```python
from build123d import *
from build123d.topology import SkipClean

# Parameters (mm, degrees)
BOSS_EXTRUDE1_DEPTH                      = 3
MIRROR1_AT_THE_SECOND_PLANE_COPY_1_DEPTH = 3
SKETCH2_R                                = 1.6
CUT_EXTRUDE1_DEPTH                       = 108.522090753
CHAMFER1_SIZE                            = 1.5
CIRPATTERN1_COUNT                        = 6
CHAMFER1_OF_CIRPATTERN1_SIZE             = 1.5
SKETCH3_R                                = 5
CUT_EXTRUDE2_DEPTH                       = 108.522090753


with BuildPart() as part:
    # Sketch1 → Boss-Extrude1 (new body)
    with BuildSketch(Plane(origin=(0, 0, 0), x_dir=(1, 0, 0), z_dir=(0, 1, 0))):
        with BuildLine():
            Line((-76, -76), (-59.111111111, -76))
            Line((-59.111111111, -76), (-59.111111111, -73))
            Line((-59.111111111, -73), (-42.222222222, -73))
            Line((-42.222222222, -73), (-42.222222222, -76))
            Line((-42.222222222, -76), (-25.333333333, -76))
            Line((-25.333333333, -76), (-25.333333333, -73))
            Line((-25.333333333, -73), (-8.444444444, -73))
            Line((-8.444444444, -73), (-8.444444444, -76))
            Line((-8.444444444, -76), (0, -76))
            Line((0, -76), (0, -10.5))
            ThreePointArc((0, -10.5), (-7.424621202, -7.424621202), (-10.5, 0))
            Line((-10.5, 0), (-76, 0))
            Line((-76, 0), (-76, -8.444444444))
            Line((-76, -8.444444444), (-73, -8.444444444))
            Line((-73, -8.444444444), (-73, -25.333333333))
            Line((-73, -25.333333333), (-76, -25.333333333))
            Line((-76, -25.333333333), (-76, -42.222222222))
            Line((-76, -42.222222222), (-73, -42.222222222))
            Line((-73, -42.222222222), (-73, -59.111111111))
            Line((-73, -59.111111111), (-76, -59.111111111))
            Line((-76, -59.111111111), (-76, -76))
        make_face()
    boss_extrude1 = extrude(amount=BOSS_EXTRUDE1_DEPTH)

    # Mirror1 at the second plane: Boss-Extrude1 across plane
    add(boss_extrude1.mirror(Plane(origin=(0, 0, 0), x_dir=(0, 0, 1), z_dir=(1, 0, 0))))



with BuildPart() as mirror1_1:
    # Mirror1: Boss-Extrude1 across plane
    add(boss_extrude1.mirror(Plane.XY))


with BuildPart() as part_1:
    with SkipClean():  # the faces are left unmerged after this step: merging them gives an invalid solid
        add(part.part)

        add(mirror1_1.part)  # Mirror1 at the second plane copy 1 merges Mirror1_1
        # Mirror1 at the second plane copy 1 sketc → Mirror1 at the second plane copy 1 (add)
        with BuildSketch(Plane(origin=(0, 0, 0), x_dir=(-1, 0, 0), z_dir=(0, 1, 0))):
            with BuildLine():
                Line((-76, -76), (-59.111111111, -76))
                Line((-59.111111111, -76), (-59.111111111, -73))
                Line((-59.111111111, -73), (-42.222222222, -73))
                Line((-42.222222222, -73), (-42.222222222, -76))
                Line((-42.222222222, -76), (-25.333333333, -76))
                Line((-25.333333333, -76), (-25.333333333, -73))
                Line((-25.333333333, -73), (-8.444444444, -73))
                Line((-8.444444444, -73), (-8.444444444, -76))
                Line((-8.444444444, -76), (0, -76))
                Line((0, -76), (0, -10.5))
                ThreePointArc((0, -10.5), (-7.424621202, -7.424621202), (-10.5, 0))
                Line((-10.5, 0), (-76, 0))
                Line((-76, 0), (-76, -8.444444444))
                Line((-76, -8.444444444), (-73, -8.444444444))
                Line((-73, -8.444444444), (-73, -25.333333333))
                Line((-73, -25.333333333), (-76, -25.333333333))
                Line((-76, -25.333333333), (-76, -42.222222222))
                Line((-76, -42.222222222), (-73, -42.222222222))
                Line((-73, -42.222222222), (-73, -59.111111111))
                Line((-73, -59.111111111), (-76, -59.111111111))
                Line((-76, -59.111111111), (-76, -76))
            make_face()
        extrude(amount=MIRROR1_AT_THE_SECOND_PLANE_COPY_1_DEPTH)

    # Sketch2 → Cut-Extrude1 (cut, through all)
    with SkipClean():  # the faces are left unmerged after this step: merging them gives an invalid solid
        with BuildSketch(Plane(origin=(0, 3, 0), x_dir=(1, 0, 0), z_dir=(0, 1, 0))):
            with Locations(Location((0, 21, 0), (0, 0, 270))):
                Circle(SKETCH2_R)
        cut_extrude1 = extrude(amount=-CUT_EXTRUDE1_DEPTH, mode=Mode.SUBTRACT)

    # Chamfer1
    chamfer1_edges = [part_1.edges().sort_by_distance(p)[0] for p in [
        (-1.6, 0, -21),
    ]]
    chamfer(chamfer1_edges, length=CHAMFER1_SIZE)

    # CirPattern1: Cut-Extrude1 ×6 about axis
    cirpattern1_axis = Axis((0, 0, 0), (0, 1, 0))
    for i in range(1, CIRPATTERN1_COUNT):
        add(cut_extrude1.rotate(cirpattern1_axis, i * 360 / CIRPATTERN1_COUNT), mode=Mode.SUBTRACT)

    # Chamfer1 of CirPattern1
    chamfer1_of_cirpattern1_edges = [part_1.edges().sort_by_distance(p)[0] for p in [
        (-18.986533479, 0, -9.114359354),
        (-17.386533479, 0, 11.885640646),
        (1.6, 0, 21),
        (18.986533479, 0, 9.114359354),
        (17.386533479, 0, -11.885640646),
    ]]
    chamfer(chamfer1_of_cirpattern1_edges, length=CHAMFER1_OF_CIRPATTERN1_SIZE)

    # Sketch3 → Cut-Extrude2 (cut, through all)
    with BuildSketch(Plane(origin=(0, 3, 0), x_dir=(1, 0, 0), z_dir=(0, 1, 0))):
        with Locations(Location((0, 42.5, 0), (0, 0, 270))):
            Circle(SKETCH3_R)
        with BuildLine():
            ThreePointArc((-21.372688022, 25.470977734), (-21.865715356, 19.835649522), (-16.230387145, 19.342622189))
            ThreePointArc((-16.230387145, 19.342622189), (0, 25.25), (16.230387145, 19.342622189))
            ThreePointArc((16.230387145, 19.342622189), (21.865715356, 19.835649522), (21.372688022, 25.470977734))
            ThreePointArc((21.372688022, 25.470977734), (0, 33.25), (-21.372688022, 25.470977734))
        make_face()
    cut_extrude2 = extrude(amount=-CUT_EXTRUDE2_DEPTH, mode=Mode.SUBTRACT)

    # Mirror2: Cut-Extrude2 across plane
    add(cut_extrude2.mirror(Plane.XY), mode=Mode.SUBTRACT)


solid = part_1.part
```
The model under review builds one solid part; all positions refer to its coordinate system, in mm. A direction names the side the tool comes from. Round coordinates to 2 decimals unless told otherwise and drop trailing zeros. Loops run counter-clockwise (first coordinate to the right, second up) from the corner with the lowest first, then second, coordinate; pieces in that order, holes last. Notation, with made-up numbers: (53.25, 11.25) -> (81.25, 11.25) arc R19 cw to (81.25, 27.25) -> close; hole circle Ø9 at (46, 72). An arc over 180 degrees is marked (long way). Answer as a JSON object with one key per item and string values. Group by question number.
1) We need section C-C on y = 2. Give the number of separate pieces and of enclosed holes in the cut face, then the cut area to 3 significant figures.
2) For faces 1 (the face through (-0.25, 1.52, 25.25)), 2 (the face through (1, 3, 18)), list the 3-axis set-ups (+Z, -Z, +X, -X, +Y, -Y) from which the entire face can be reached by the end or side of a thin tool; tool diameter is ignored.
3) We need section B-B on z = 16. Write out the cut boundary in (x, y), then the cut area to 3 significant figures.
4) Mouldability with a two-part tool opening along X and no side actions: class faces 3 (the face through (-21.92, 1.52, -19.9)), 4 (the face through (18, 0, 1)) as released by +X, released by -X, zero draft, split by the parting line, or undercut.
5) For line 1 (Z direction, x = -12, y = 1.95); line 2 (Z direction, x = 17, y = 2.3); line 3 (X direction, y = 2.2, z = 21), list the stretches that pass through material, from the lowest coordinate up. Write a range as [from, to].
6) We need section A-A on z = -44. Write out the cut boundary in (x, y), then the cut area to 3 significant figures.
7) For pin 1 Ø0.9 at (x, y) = (17, 2) entering from +Z; pin 2 Ø1 at (y, z) = (2.5, 51) entering from +X; pin 3 Ø1.9 at (x, z) = (18.19, 10.5) entering from +Y; pin 4 Ø0.9 at (y, z) = (2, -17.5) entering from -X, all flat-tipped, find the tip position at first contact; note any pin that passes through.
Result set:
{
 "1": {"separate pieces": "1", "enclosed holes": "11", "area": "21,000 mm²"},
 "2": {"face 1": "+Y, -Y", "face 2": "+Z, -Z, +X, -X, +Y"},
 "3": {"outline": "(-73, 0) -> (73, 0) -> (73, 3) -> (-73, 3) -> close", "area": "438 mm²"},
 "4": {"face 3": "undercut", "face 4": "zero draft"},
 "5": {"line 1": "[-73, -31.01], [-22.22, 22.22], [31.01, 73]", "line 2": "[-73, -28.58], [-18.84, -11.57], [-9.43, 9.43], [11.57, 18.84], [28.58, 73]", "line 3": "[-73, -22.55], [-14.02, -1.6], [1.6, 14.02], [22.55, 73]"},
 "6": {"outline": "(-73, 0) -> (-4.77, 0) -> (-4.77, 3) -> (-73, 3) -> close; (4.77, 0) -> (73, 0) -> (73, 3) -> (4.77, 3) -> close", "area": "409 mm²"},
 "7": {"pin 1": "z = 73", "pin 2": "x = 73", "pin 3": "through", "pin 4": "x = -73"}
}
